Verification items for this drawing (mm, ordinates from the low corner). Round coordinates to 2 decimals unless told otherwise and drop trailing zeros. Loops run counter-clockwise (first coordinate to the right, second up) from the corner with the lowest first, then second, coordinate; pieces in that order, holes last. Notation, with made-up numbers: M -21.5,9.25 L -17.5,9.25 A27 cw -17.5,28.25 Z; hole C 21.25,-11.75 d9. An arc over 180 degrees is marked long. Write item = value, one per line. Start each with the question number.
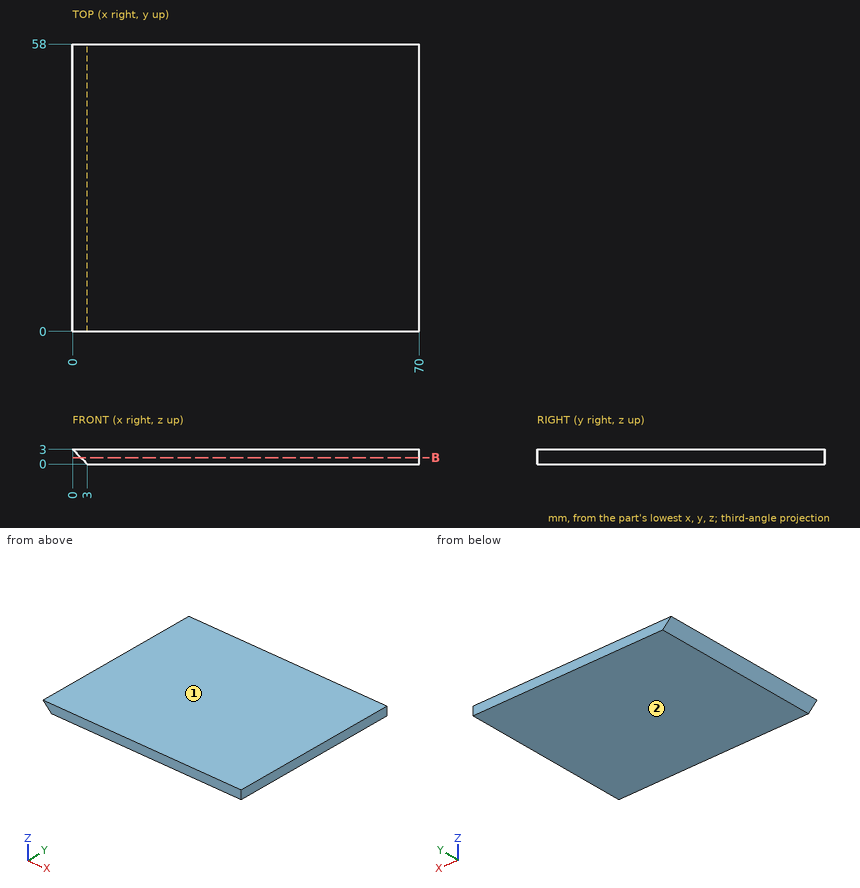
1. Section check B-B, the plane z = 1.3. Enter the section's corners in (x, y).
2. Thickness scan on line 1 (X direction, y = 34, z = 2.05); line 2 (X direction, y = 32.5, z = 0.95). Record the ranges inside material, lowest first.
3. Mould release check, pull along Z, two halves, no side actions. Record for the marked faces 1 and 2: pulls with the +Z half, pulls with the -Z half, needs draft (parallel to the pull), parting line crosses it, or undercut.
Computed values:
q1.outline = M 1.7,0 L 70,0 L 70,58 L 1.7,58 Z
q2.line_1 = 0.95 to 70
q2.line_2 = 2.05 to 70
q3.face_1 = pulls with the +Z half
q3.face_2 = pulls with the -Z half
